```python
from build123d import *

# Parameters (mm, degrees)
BOSS_EXTRUDE1_DEPTH = 6.35
CUT_EXTRUDE1_DEPTH  = 127


with BuildPart() as part:
    # Sketch1 → Boss-Extrude1 (new, symmetric)
    with BuildSketch(Plane.XY):
        Polygon((114.3, -165.1), (-114.3, -165.1), (-114.3, 165.1), (-31.75, 165.1), (-31.75, 114.3), (31.75, 114.3), (31.75, 165.1), (114.3, 165.1), align=None)
    extrude(amount=BOSS_EXTRUDE1_DEPTH, both=True)

    # Sketch2 → Cut-Extrude1 (cut, symmetric)
    with BuildSketch(Plane(origin=(0, 0, 0), x_dir=(0, 0, -1), z_dir=(1, 0, 0))):
        Polygon((-6.35, 165.1), (6.35, 165.1), (6.35, 157.767651581), align=None)
    extrude(amount=CUT_EXTRUDE1_DEPTH, both=True, mode=Mode.SUBTRACT)


solid = part.part
```
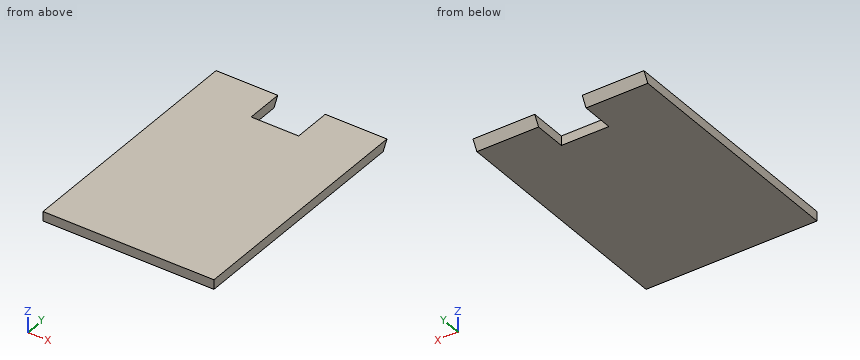
Could you check a few things on this model? Use its own coordinates, in mm. Round coordinates to 2 decimals unless told otherwise and drop trailing zeros. Loops run counter-clockwise (first coordinate to the right, second up) from the corner with the lowest first, then second, coordinate; pieces in that order, holes last. Notation, with made-up numbers: M -39.75,17 L -0.75,17 A26 ccw -0.75,55 Z; hole C -23,16.5 d8. An arc over 180 degrees is marked long. Put each result on its own line as item: value.
Q1. Imagine slicing it at A-A (z = 0). Write out the boundary of the cut face in (x, y).
Check result:
outline: M -114.3,-165.1 L 114.3,-165.1 L 114.3,161.43 L 31.75,161.43 L 31.75,114.3 L -31.75,114.3 L -31.75,161.43 L -114.3,161.43 Z
Q2. Imagine slicing it at B-B (x = -3). Write out the boundary of the cut face in (y, z), then the cut area to 3 significant figures.
Check result:
outline: M -165.1,-6.35 L 114.3,-6.35 L 114.3,6.35 L -165.1,6.35 Z
area: 3,550 mm2
Q3. I need wall thicknesses on probe 1 along X at (y, z) = (126.5, 2.5); probe 2 along Y at (x, z) = (21, 3.75); probe 3 along Y at (x, z) = (53.5, 0). Which ranges of each line are inside material? Lowest first, please.
Check result:
probe 1: -114.3 to -31.75, 31.75 to 114.3
probe 2: -165.1 to 114.3
probe 3: -165.1 to 161.43
Q4. For pin 1 (3 mm diameter, centred on x = -68, z = 0, fed in from +Y), with a flat end and sliding along its axis, tell me the tip position at first contact or that it passes through.
Check result:
pin 1: y = 162.3
